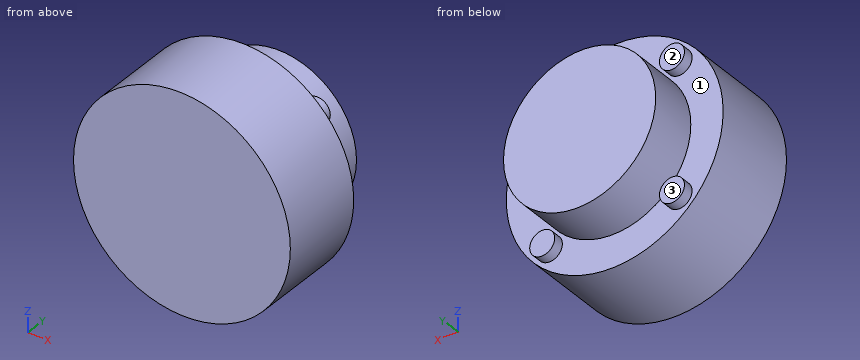
from build123d import *

# Parameters (mm, degrees)
SKETCH4_R           = 3
BOSS_EXTRUDE1_DEPTH = 2.5


with BuildPart() as part:
    # Sketch3 → Revolve1 (revolve)
    with BuildSketch(Plane.XY):
        Polygon((0, 0), (26, 0), (26, 20.758), (18.25, 20.758), (18.25, 32.258), (0, 32.258), align=None)
    revolve(axis=Axis((0, 32.258, 0), (0, -1, 0)))

    # Sketch4 → Boss-Extrude1 (add)
    with BuildSketch(Plane(origin=(0, 20.758, 0), x_dir=(1, 0, 0), z_dir=(0, 1, 0))):
        with Locations((-15.556349186, 15.556349186)):
            Circle(SKETCH4_R)
        with Locations((15.556349186, 15.556349186)):
            Circle(SKETCH4_R)
        with Locations((15.556349186, -15.556349186)):
            Circle(SKETCH4_R)
        with Locations((-15.556349186, -15.556349186)):
            Circle(SKETCH4_R)
    extrude(amount=BOSS_EXTRUDE1_DEPTH)


solid = part.part
Design review of the part built by this model. Coordinates are the model's own, in mm. Face numbers are marked on the shaded views. A direction names the side the tool comes from. Round coordinates to 2 decimals unless told otherwise and drop trailing zeros. Write each loop counter-clockwise with the first axis right and the second up, starting at its lowest first coordinate (ties: lowest second). Pieces come first, ordered by that corner, then holes.
Item 1: Consider section A-A on z = 0. Give the boundary of the cut face in (x, y).
Item 2: Consider section D-D on x = 14. Give the boundary of the cut face in (y, z), and give its area (3 significant figures).
Item 3: Consider section B-B on x = 0. Give the boundary of the cut face in (y, z).
Item 4: For pin 1 Ø3 at (y, z) = (8, 13) entering from +X; pin 2 Ø8 at (x, y) = (1.5, 23.5) entering from +Z; pin 3 Ø1.5 at (x, z) = (12.5, 20) entering from +Y, all flat-tipped, find the tip position at first contact; note any pin that passes through.
Item 5: Wall thickness on L1, parallel to Y at x = -21, z = -3; L2, parallel to Z at x = -3.5, y = 30; L3, parallel to Y at x = 14.5, z = 16.5: over which ranges is each line inside the solid? List them lowest first.
Item 6: For the marked faces 1, 2 and 3, list the 3-axis set-ups (+Z, -Z, +X, -X, +Y, -Y) from which the entire face can be reached by the end or side of a thin tool; tool diameter is ignored.
Item 7: Consider section C-C on y = 3. Give the boundary of the cut face in (x, z), and give its area (3 significant figures).
Check values:
1. outline: (-26, 0) - (26, 0) - (26, 20.76) - (18.25, 20.76) - (18.25, 32.26) - (-18.25, 32.26) - (-18.25, 20.76) - (-26, 20.76) - close
2. outline: (0, -21.91) - (20.76, -21.91) - (20.76, -18.12) - (23.26, -18.12) - (23.26, -12.99) - (20.76, -12.99) - (20.76, -11.71) - (32.26, -11.71) - (32.26, 11.71) - (20.76, 11.71) - (20.76, 12.99) - (23.26, 12.99) - (23.26, 18.12) - (20.76, 18.12) - (20.76, 21.91) - (0, 21.91) - close
2. area: 1,200 mm2
3. outline: (0, -26) - (20.76, -26) - (20.76, -18.25) - (32.26, -18.25) - (32.26, 18.25) - (20.76, 18.25) - (20.76, 26) - (0, 26) - close
4. pin 1: stops at x = 23.32
4. pin 2: stops at z = 26
4. pin 3: stops at y = 20.76
5. L1: y = 0 to 20.76
5. L2: z = -17.91 to 17.91
5. L3: y = 0 to 23.26
6. face 1: +Y
6. face 2: +Z, -X, +Y
6. face 3: -Z, -X, +Y
7. outline: circle Ø52 at (0, 0)
7. area: 2,120 mm2
